Geometry check sheet. Reference: the model listing, model coordinates, mm. A direction names the side the tool comes from. Round coordinates to 2 decimals unless told otherwise and drop trailing zeros. Order: outer loops, then holes, each group sorted by start corner. A loop starts at its lowest first (then second) coordinate and runs counter-clockwise, first axis right, second up. Notation, with made-up numbers: (37.5, 8.25) - (52.5, 8.25) arc R20 cw to (52.5, 30.25) - close; hole circle Ø8 at (-25, -10). An arc over 180 degrees is marked (long way). One line per question, with ' | ' between items. Start each with the question number.
Q1. Tool access check on faces 5 (the face through (15.621, 0, 2)), 6 (the face through (66, 12, 0)). Record the directions out of +Z, -Z, +X, -X, +Y, -Y that give a thin tool (end or side, any length) a straight path to the whole face; none if there is none.
Q2. Sectioned sample at D-D, the plane x = 102. Enter the section's corners in (y, z), then the cut area to 3 significant figures.
Q3. Gauge pin test, flat ends, axial feed: P1, Ø2, axis at x = 39, y = 12.5, coming from the -Z side; P2, Ø1, axis at y = 14, z = 2, coming from the -X side; P3, Ø1.4, axis at x = -16, z = 1.5, coming from the -Y side (3 decimals); P4, Ø1, axis at x = 125.5, z = 1, coming from the -Y side. Record the tip position at first contact, or that the pin passes through.
Q4. Sectioned sample at A-A, the plane y = 7.5. Enter the section's corners in (x, z) (3 decimals).
Q5. Sectioned sample at B-B, the plane z = 1.55. Enter the section's corners in (x, y) (1 decimal), then the cut area to 3 significant figures.
Q6. Mould release check, pull along X, two halves, no side actions. Record for faces 1 (the face through (115.75, 18.68, 1.63)), 2 (the face through (114.48, 0.83, 1.63)), 3 (the face through (-18.404, 15.211, 1.628)), 4 (the face through (-17.167, -3.53, 1.628)): +X half, -X half, draft (parallel to the pull), parting line (faces both ways), or undercut.
Q7. Sectioned sample at C-C, the plane x = 143. Enter the section's corners in (y, z).
Q8. Material ranges on line 1 along X through (y, z) = (8.5, 2.65); line 2 along X through (y, z) = (10, 1.2); line 3 along Y through (x, z) = (-0.5, 2.8), recorded low to high.
```python
from build123d import *

# Parameters (mm, degrees)
F0_R     = 5.196102
F1_DEPTH = 3.302
F2_R     = 5.08


with BuildPart() as f1:
    # F0 (on Top) → F1 (new body)
    with BuildSketch(Plane.XY):
        with BuildLine():
            ThreePointArc((17.42216, -1.905), (17.171429, -3.507522), (16.773618, -5.08))
            ThreePointArc((16.773618, -5.08), (20.051467, -8.357849), (23.329316, -5.08))
            Line((23.329316, -5.08), (79.846062, 3.404097))
            Line((79.846062, 3.404097), (149.504127, -1.770501))
            ThreePointArc((149.504127, -1.770501), (157.802675, 5.538416), (150.315792, 13.676766))
            Line((150.315792, 13.676766), (79.846062, 23.876))
            Line((79.846062, 23.876), (0, 23.876))
            ThreePointArc((0, 23.876), (-18.592384, 14.979541), (-23.329316, -5.08))
            ThreePointArc((-23.329316, -5.08), (-20.051467, -8.357849), (-16.773618, -5.08))
            ThreePointArc((-16.773618, -5.08), (-17.171429, -3.507522), (-17.42216, -1.905))
            ThreePointArc((-17.42216, -1.905), (-17.526, 0), (-17.42216, 1.905))
            ThreePointArc((-17.42216, 1.905), (-12.392753, 12.392753), (-1.905, 17.42216))
            ThreePointArc((-1.905, 17.42216), (0, 17.526), (1.905, 17.42216))
            ThreePointArc((1.905, 17.42216), (12.392753, 12.392753), (17.42216, 1.905))
            ThreePointArc((17.42216, 1.905), (17.526, 0), (17.42216, -1.905))
        make_face()
        with Locations((150.07723, 5.944343)):
            Circle(F0_R, mode=Mode.SUBTRACT)
        with BuildLine():
            Line((1.905, 15.621), (1.905, 17.42216))
            ThreePointArc((1.905, 17.42216), (0, 17.526), (-1.905, 17.42216))
            Line((-1.905, 17.42216), (-1.905, 15.621))
            Line((-1.905, 15.621), (1.905, 15.621))
        make_face()
        with BuildLine():
            Line((15.621, -1.905), (17.42216, -1.905))
            ThreePointArc((17.42216, -1.905), (17.526, 0), (17.42216, 1.905))
            Line((17.42216, 1.905), (15.621, 1.905))
            Line((15.621, 1.905), (15.621, -1.905))
        make_face()
        with BuildLine():
            Line((-15.621, 1.905), (-17.42216, 1.905))
            ThreePointArc((-17.42216, 1.905), (-17.526, 0), (-17.42216, -1.905))
            Line((-17.42216, -1.905), (-15.621, -1.905))
            Line((-15.621, -1.905), (-15.621, 1.905))
        make_face()
    extrude(amount=F1_DEPTH)

    # F2
    f2_edges = [f1.edges().sort_by_distance(p)[0] for p in [
        (23.329316, -5.08, 1.651),
        (79.846062, 3.404097, 1.651),
        (79.846062, 23.876, 1.651),
    ]]
    fillet(f2_edges, radius=F2_R)


solid = f1.part
```
Determined:
1) face 5: +Z, -Z, -Y | face 6: -Z, +X, -X, +Y, -Y
2) outline: (1.76, 0) - (20.67, 0) - (20.67, 3.3) - (1.76, 3.3) - close | area: 62.4 mm2
3) P1: stops at z = 0 | P2: stops at x = -19.69 | P3: stops at y = -1.905 | P4: stops at y = -0.02
4) outline: (-22.667, 0) - (-15.84, 0) - (-15.84, 3.302) - (-22.667, 3.302) - close; (15.84, 0) - (145.119, 0) - (145.119, 3.302) - (15.84, 3.302) - close; (155.035, 0) - (157.655, 0) - (157.655, 3.302) - (155.035, 3.302) - close
5) outline: (-23.3, -5.1) arc R3.3 ccw to (-16.8, -5.1) arc R17.5 cw to (-17.4, -1.9) - (-15.6, -1.9) - (-15.6, 1.9) - (-17.4, 1.9) arc R17.5 cw to (-1.9, 17.4) - (-1.9, 15.6) - (1.9, 15.6) - (1.9, 17.4) arc R17.5 cw to (17.4, 1.9) - (15.6, 1.9) - (15.6, -1.9) - (17.4, -1.9) arc R17.5 cw to (16.8, -5.1) arc R3.3 ccw to (22.8, -6.9) arc R5.1 cw to (26.3, -4.6) - (79.3, 3.3) arc R5.1 cw to (80.4, 3.4) - (149.5, -1.8) arc R7.7 ccw (long way) to (150.3, 13.7) - (80.2, 23.8) arc R5.1 ccw to (79.5, 23.9) - (0, 23.9) arc R23.9 ccw to start; hole circle Ø10.4 at (150.1, 5.9) | area: 3,310 mm2
6) face 1: +X half | face 2: undercut | face 3: -X half | face 4: undercut
7) outline: (-1.29, 0) - (14.74, 0) - (14.74, 3.3) - (-1.29, 3.3) - close
8) line 1: x = -22.31 to -15.33, 15.33 to 145.55, 154.6 to 157.38 | line 2: x = -21.68 to -14.39, 14.39 to 146.83, 153.33 to 156.67 | line 3: y = 15.62 to 23.87
